The listing builds one solid part. Answer for the finished solid, in the listing's coordinates (mm). Coordinates: 2 decimals unless noted, no trailing zeros. Loops run counter-clockwise (first coordinate to the right, second up) from the corner with the lowest first, then second, coordinate; pieces in that order, holes last. Notation, with made-up numbers: M 36.25,51 L 83.25,51 A18 ccw 83.25,58 Z; hole C -20,52 d9. An arc over 180 degrees is marked long. Return JSON: item names as keys, results as strings. Group by question number.
1. Given P1, Ø6, axis at x = 24, y = -24.5, coming from the -Z side; P2, Ø4, axis at x = 16.5, z = 7.5, coming from the +Y side; P3, Ø1, axis at x = -16.5, z = 1, coming from the -Y side; P4, Ø1.5, axis at y = -3, z = -1, coming from the +X side, each flat-ended and moving along its own axis, determine where each tip first touches the part or whether it passes through.
2. Straight lines are drawn through the part: L1, parallel to Y at x = 0, z = 8.1; L2, parallel to Z at x = 4.5, y = 16; L3, parallel to X at y = -3, z = 0.5. For each, find the intervals that lie inside material, in ascending order. Write a range as from..to.
3. Section D-D (x = -23) is taken. Write down the section's boundary in (y, z), then the cut area to 3 significant figures.
4. Section A-A (x = 0) is taken. Write down the section's boundary in (y, z), then the cut area to 4 significant figures.
5. Section C-C (z = 2.5) is taken. Write down the section's boundary in (x, y).
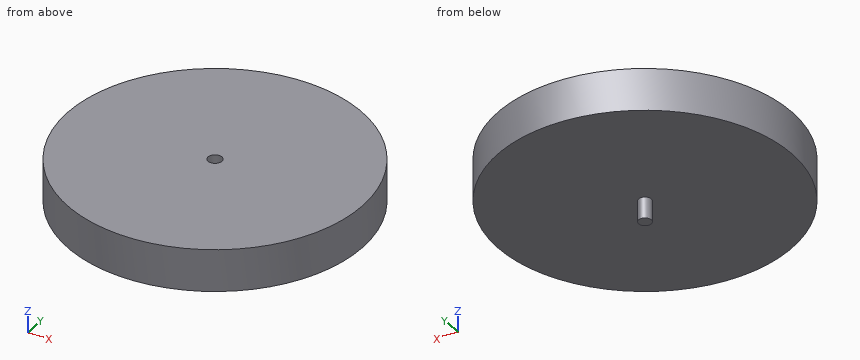
```python
from build123d import *

# Parameters (mm, degrees)
SKETCH1_R           = 35
BOSS_EXTRUDE1_DEPTH = 10
SKETCH2_R           = 1.5
BOSS_EXTRUDE2_DEPTH = 5
SKETCH3_R           = 1.65
CUT_EXTRUDE1_DEPTH  = 5


with BuildPart() as part:
    # Sketch1 → Boss-Extrude1 (new body)
    with BuildSketch(Plane.XY):
        Circle(SKETCH1_R)
    extrude(amount=BOSS_EXTRUDE1_DEPTH)

    # Sketch2 → Boss-Extrude2 (add)
    with BuildSketch(Plane(origin=(0, 0, 0), x_dir=(-1, 0, 0), z_dir=(0, 0, -1))):
        Circle(SKETCH2_R)
    extrude(amount=BOSS_EXTRUDE2_DEPTH)

    # Sketch3 → Cut-Extrude1 (cut)
    with BuildSketch(Plane.XY.offset(10)):
        Circle(SKETCH3_R)
    extrude(amount=-CUT_EXTRUDE1_DEPTH, mode=Mode.SUBTRACT)


solid = part.part
```
Worked out:
{
 "1": {"P1": "z = 0", "P2": "y = 31.86", "P3": "y = -31.13", "P4": "through"},
 "2": {"L1": "-35..-1.65, 1.65..35", "L2": "0..10", "L3": "-34.87..34.87"},
 "3": {"outline": "M -26.38,0 L 26.38,0 L 26.38,10 L -26.38,10 Z", "area": "528 mm^2"},
 "4": {"outline": "M -35,0 L -1.5,0 L -1.5,-5 L 1.5,-5 L 1.5,0 L 35,0 L 35,10 L 1.65,10 L 1.65,5 L -1.65,5 L -1.65,10 L -35,10 Z", "area": "698.5 mm^2"},
 "5": {"outline": "C 0,0 d70"}
}
